from build123d import *

# Parameters (mm, degrees)
BOSS_EXTRUDE1_DEPTH = 1524
BOSS_EXTRUDE2_DEPTH = 1524
FILLET1_R           = 0.75
FILLET2_R           = 1.25
SKETCH5_W           = 1548
SKETCH5_H           = 20
CUT_EXTRUDE1_DEPTH  = 1525.55764076


with BuildPart() as part:
    # Sketch3 → Boss-Extrude1 (new, symmetric)
    with BuildSketch(Plane.XY):
        with BuildLine():
            Line((12.5, -10), (17.9, -10))
            ThreePointArc((17.9, -10), (19.38492424, -9.38492424), (20, -7.9))
            Line((20, -7.9), (20, -2.5))
            Line((20, -2.5), (18.213351365, -2.5))
            Line((18.213351365, -2.5), (18.213351365, -6.95))
            Line((18.213351365, -6.95), (13.6, -2.336648635))
            Line((13.6, -2.336648635), (13.6, 0))
            Line((13.6, 0), (12.15, 0))
            ThreePointArc((12.15, 0), (11.52027958, -1.52027958), (10, -2.15))
            Line((10, -2.15), (10, -3.6))
            Line((10, -3.6), (12.336648635, -3.6))
            Line((12.336648635, -3.6), (16.95, -8.213351365))
            Line((16.95, -8.213351365), (12.5, -8.213351365))
            Line((12.5, -8.213351365), (12.5, -10))
        make_face()
    extrude(amount=BOSS_EXTRUDE1_DEPTH, both=True)

    # Sketch4 → Boss-Extrude2 (add, symmetric)
    with BuildSketch(Plane.XY):
        with BuildLine():
            Line((10, -3.6), (7.663351365, -3.6))
            Line((7.663351365, -3.6), (3.05, -8.213351365))
            Line((3.05, -8.213351365), (7.5, -8.213351365))
            Line((7.5, -8.213351365), (7.5, -10))
            Line((7.5, -10), (0, -10))
            Line((0, -10), (0, -8.736648635))
            Line((0, -8.736648635), (6.4, -2.336648635))
            Line((6.4, -2.336648635), (6.4, 0))
            Line((6.4, 0), (7.85, 0))
            ThreePointArc((7.85, 0), (8.47972042, -1.52027958), (10, -2.15))
            Line((10, -2.15), (10, -3.6))
        make_face()
    extrude(amount=BOSS_EXTRUDE2_DEPTH, both=True)

    # Mirror1: part across plane


with BuildPart() as part_1:
    add(part.part)
    add(part.part.mirror(Plane(origin=(0, 0, 0), x_dir=(0, 0, 1), z_dir=(1, 0, 0))))

    # Mirror2: part across plane


with BuildPart() as part_2:
    add(part_1.part)
    add(part_1.part.mirror(Plane.ZX))

    # Fillet1
    fillet1_edges = [part_2.edges().sort_by_distance(p)[0] for p in [
        (18.213351365, 6.95, 0),
        (13.6, 2.336648635, 0),
        (12.336648635, 3.6, 0),
        (16.95, 8.213351365, 0),
        (3.05, 8.213351365, 0),
        (7.663351365, 3.6, 0),
        (-18.213351365, 6.95, 0),
        (-13.6, 2.336648635, 0),
        (-7.663351365, 3.6, 0),
        (-12.336648635, 3.6, 0),
        (-16.95, 8.213351365, 0),
        (-3.05, 8.213351365, 0),
        (16.95, -8.213351365, 0),
        (12.336648635, -3.6, 0),
        (13.6, -2.336648635, 0),
        (18.213351365, -6.95, 0),
        (3.05, -8.213351365, 0),
        (7.663351365, -3.6, 0),
        (-18.213351365, -6.95, 0),
        (-13.6, -2.336648635, 0),
        (-12.336648635, -3.6, 0),
        (-16.95, -8.213351365, 0),
        (-3.05, -8.213351365, 0),
        (-7.663351365, -3.6, 0),
    ]]
    fillet(fillet1_edges, radius=FILLET1_R)

    # Fillet2
    fillet2_edges = [part_2.edges().sort_by_distance(p)[0] for p in [
        (6.4, 2.336648635, 0),
        (0, 8.736648635, 0),
        (-6.4, 2.336648635, 0),
        (6.4, -2.336648635, 0),
        (-6.4, -2.336648635, 0),
        (0, -8.736648635, 0),
    ]]
    fillet(fillet2_edges, radius=FILLET2_R)

    # Sketch5 → Cut-Extrude1 (cut, through all)
    with BuildSketch(Plane.ZY.offset(20)):
        with Locations((750, 0)):
            Rectangle(SKETCH5_W, SKETCH5_H)
    extrude(amount=-CUT_EXTRUDE1_DEPTH, mode=Mode.SUBTRACT)


solid = part_2.part
Work out the finished part from the listing and answer in its coordinate system (mm). Give positions to 0.01 mm unless a question says otherwise; leave off trailing zeros.
Q1. The part is cut by section A-A on z = -142. State how many separate pieces and enclosed holes the cut face has, and give its area (3 significant figures).
Answer:
separate pieces: 1
enclosed holes: 3
area: 324 mm2
Q2. Given pin 1 (2 mm diameter, centred on y = -9, z = -1040.5, fed in from -X); pin 2 (1.4 mm diameter, centred on x = 19, z = -849, fed in from -Y); pin 3 (1 mm diameter, centred on x = -9, z = -1197.5, fed in from +Y); pin 4 (3 mm diameter, centred on x = -8.5, z = -275, fed in from +Y), each flat-ended and moving along its own axis, determine where each tip first touches the part or whether it passes through.
Answer:
pin 1: stops at x = -20
pin 2: stops at y = -9.96
pin 3: stops at y = 3.6
pin 4: stops at y = 10
Q3. Straight lines are drawn through the part: L1, parallel to X at y = 7.75, z = -603; L2, parallel to X at y = 6.5, z = -205; L3, parallel to Y at x = -6, z = -523.5. For each, find the intervals that lie inside material, in ascending order.
Answer:
L1: x = -20 to -15.83, -4.17 to -0.99, 0.99 to 4.17, 15.83 to 20
L2: x = -20 to -15.24, -4.76 to -2.24, 2.24 to 4.76, 15.24 to 20
L3: y = -10 to -8.21, -5.26 to -2.74, 2.74 to 5.26, 8.21 to 10
